Check sheet for the drawn part. Datum: minimum x, y, z corner. Units: mm. A direction names the side the tool comes from. Round coordinates to 2 decimals unless told otherwise and drop trailing zeros. Write each loop counter-clockwise with the first axis right and the second up, starting at its lowest first coordinate (ties: lowest second). Pieces come first, ordered by that corner, then holes. Notation, with made-up numbers: M 2.25,-6 L 12.25,-6 A30 ccw 12.25,31 Z; hole C 13,31.5 d4. An arc over 180 degrees is marked long. One line per item, written item: value. Start each with the question number.
Item 1: Draft check along Z on the marked faces 1, 2 and 3. Enter one of: +Z half, -Z half, draft (parallel to the pull), parting line (faces both ways), or undercut.
Item 2: Section check C-C, the plane y = 41. Record the cut outline in (x, z), then the cut area to 3 significant figures.
Item 3: Section check B-B, the plane x = 47. Record the cut outline in (y, z).
Item 4: Section check D-D, the plane z = 35. Record the cut outline in (x, y).
Item 5: Thickness scan on probe 1 along Z at (x, y) = (17, 108); probe 2 along X at (y, z) = (93, 18); probe 3 along X at (y, z) = (154, 46). Record the ranges inside material, lowest first. Write a range as from..to.
Item 6: Tool access check on the marked faces 4 and 5. Record the directions out of +Z, -Z, +X, -X, +Y, -Y that give a thin tool (end or side, any length) a straight path to the whole face; none if there is none.
Item 7: Gauge pin test, flat ends, axial feed: pin 1 (8 mm diameter, centred on y = 159, z = 5, fed in from +X); pin 2 (9 mm diameter, centred on x = 34, z = 34.5, fed in from +Y); pin 3 (11 mm diameter, centred on y = 157, z = 48, fed in from +X). Record the tip position at first contact, or that the pin passes through.
Item 8: Section check A-A, the plane x = 36. Record the cut outline in (y, z), then the cut area to 3 significant figures.
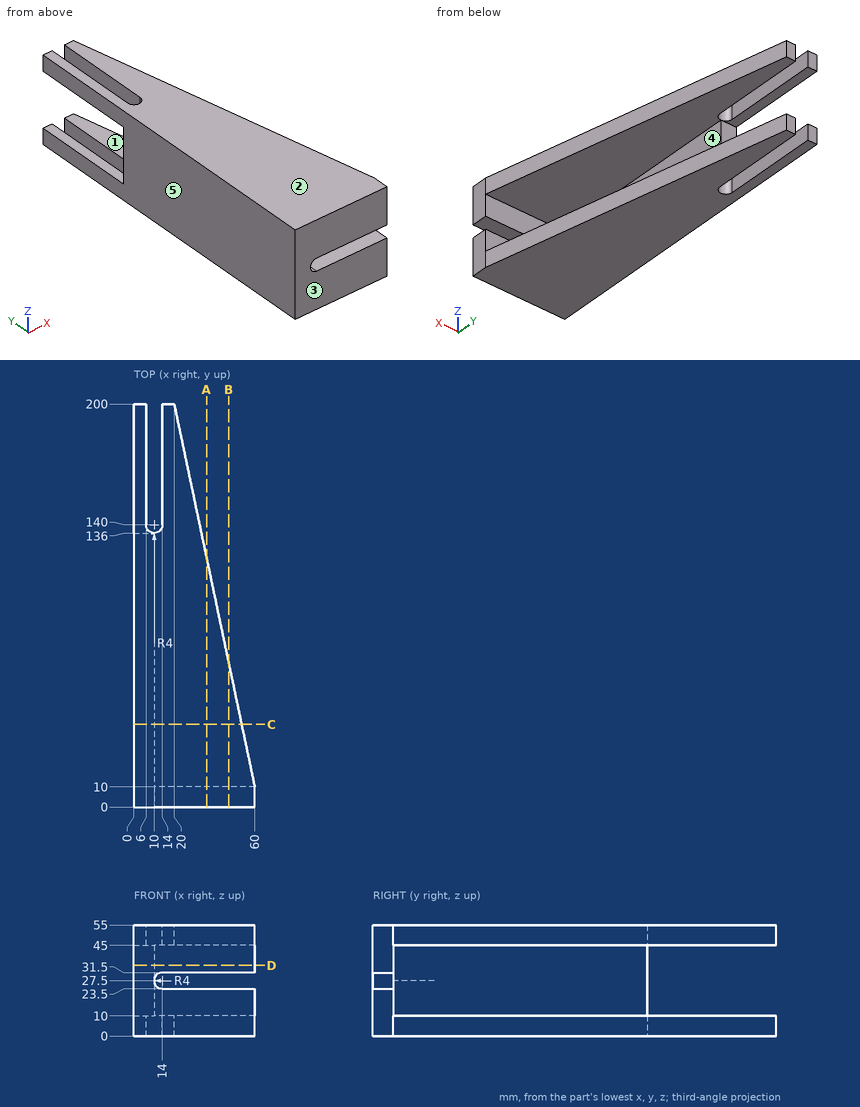
Response values:
1. face 1: undercut
1. face 2: +Z half
1. face 3: draft
2. outline: M 0,0 L 53.47,0 L 53.47,10 L 10,10 L 10,45 L 53.47,45 L 53.47,55 L 0,55 Z
2. area: 1,420 mm2
3. outline: M 0,0 L 71.75,0 L 71.75,10 L 10,10 L 10,23.5 L 0,23.5 Z; M 0,31.5 L 10,31.5 L 10,45 L 71.75,45 L 71.75,55 L 0,55 Z
4. outline: M 0,0 L 60,0 L 60,10 L 10,10 L 10,136 L 0,136 Z
5. probe 1: z = 0..10, 45..55
5. probe 2: x = 0..10
5. probe 3: x = 0..6, 14..29.68
6. face 4: +X, +Y
6. face 5: +Z, -Z, -X, +Y, -Y
7. pin 1: stops at x = 29.47
7. pin 2: stops at y = 10
7. pin 3: stops at x = 30.21
8. outline: M 0,0 L 124,0 L 124,10 L 10,10 L 10,23.5 L 0,23.5 Z; M 0,31.5 L 10,31.5 L 10,45 L 124,45 L 124,55 L 0,55 Z
8. area: 2,750 mm2
